```python
from build123d import *

# Parameters (mm, degrees)
F0_R     = 4
F0_R_2   = 2
F1_DEPTH = 8
F3_DEPTH = 1
F4_R     = 2.54


with BuildPart() as f1:
    # F0 (on Front) → F1 (new body)
    with BuildSketch(Plane.XZ):
        Circle(F0_R)
        Circle(F0_R_2, mode=Mode.SUBTRACT)
    extrude(amount=F1_DEPTH)

    # F2 (on Front) → F3 (join)
    with BuildSketch(Plane.XZ):
        Polygon((5.9944, 49.53), (-6.0056, 49.53), (-6.0056, 5.08), (-2.54, 2.54), (2.54, 2.54), (5.9944, 5.08), align=None)
        Polygon((-5.9944, -5.08), (-5.9944, -49.53), (5.9944, -49.53), (5.9944, -5.08), (2.54, -2.54), (-2.54, -2.54), align=None)
    extrude(amount=F3_DEPTH)

    # F4
    f4_edges = [f1.edges().sort_by_distance(p)[0] for p in [
        (-6.0056, -0.5, 49.53),
        (5.9944, -0.5, 49.53),
        (5.9944, -0.5, -49.53),
        (-5.9944, -0.5, -49.53),
    ]]
    fillet(f4_edges, radius=F4_R)


solid = f1.part
```
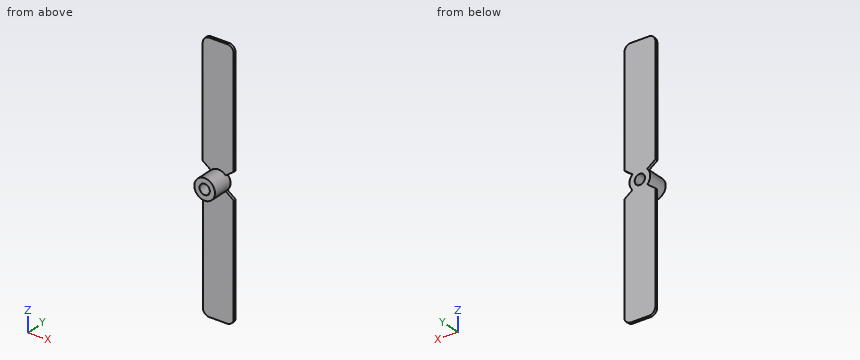
The model under review builds one solid part; all positions refer to its coordinate system, in mm. Round coordinates to 2 decimals unless told otherwise and drop trailing zeros. Loops run counter-clockwise (first coordinate to the right, second up) from the corner with the lowest first, then second, coordinate; pieces in that order, holes last.
Item 1: Take a section at D-D (z = 30). Write out the cut boundary in (x, y).
Determined:
outline: (-6.01, -1) - (5.99, -1) - (5.99, 0) - (-6.01, 0) - close
Item 2: For line 1 (Z direction, x = 0, y = -4.75); line 2 (Y direction, x = -3.5, z = 16); line 3 (Z direction, x = -1.25, y = -2.5), list the stretches that pass through material, from the lowest coordinate up.
Determined:
line 1: z = -4 to -2, 2 to 4
line 2: y = -1 to 0
line 3: z = -3.8 to -1.56, 1.56 to 3.8
Item 3: Take a section at A-A (x = 0). Write out the cut boundary in (y, z).
Determined:
outline: (-8, -4) - (-1, -4) - (-1, -49.53) - (0, -49.53) - (0, -2) - (-8, -2) - close; (-8, 2) - (0, 2) - (0, 49.53) - (-1, 49.53) - (-1, 4) - (-8, 4) - close
Item 4: Take a section at B-B (z = 0). Write out the cut boundary in (x, y).
Determined:
outline: (-4, -8) - (-2, -8) - (-2, 0) - (-4, 0) - close; (2, -8) - (4, -8) - (4, 0) - (2, 0) - close
Item 5: Clearance check with flat-ended pins moving along their axes: pin 1 Ø4 at (y, z) = (-1.5, 3) entering from -X; pin 2 Ø5 at (x, z) = (0.5, -32) entering from +Y; pin 3 Ø3.5 at (x, z) = (-2.5, 27.5) entering from -Y. State where each tip first meets the part, or that it passes through.
Determined:
pin 1: stops at x = -5.81
pin 2: stops at y = 0
pin 3: stops at y = -1
Item 6: Take a section at C-C (y = -2.75). Write out the cut boundary in (x, z), then the cut area to 3 significant figures.
Determined:
outline: circle Ø8 at (0, 0); hole circle Ø4 at (0, 0)
area: 37.7 mm2
